Geometry: see drawing. Coordinates: mm, zero at the bounding-box minimum. Give positions to 0.01 mm unless a question says otherwise; leave off trailing zeros. Write each loop counter-clockwise with the first axis right and the second up, starting at its lowest first coordinate (ties: lowest second). Pieces come first, ordered by that corner, then holes.
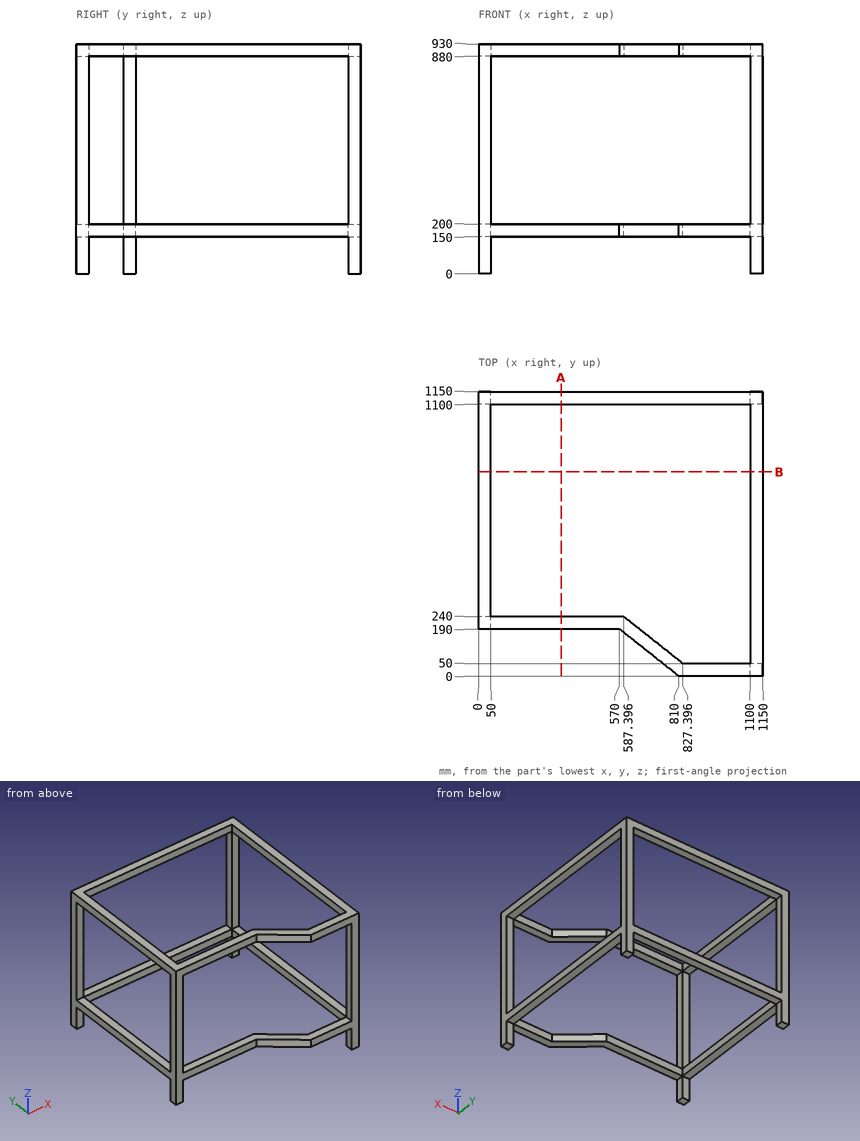
1. Line query: probe 1 along X at (y, z) = (209, 713); probe 2 along Y at (x, z) = (346, 172); probe 3 along Y at (x, z) = (624, 880.5). Output: solid intervals per line, ascending.
2. Pin query (flat end, axial travel): P1, Ø25, axis at x = 17, z = 79, coming from the -Y side. Return the tip coordinate at first contact, or that it passes through.
3. Section query B-B (y = 826.5). Return loops of the section in (x, z), plus the area to 3 significant figures.
4. Section query A-A (x = 334). Return loops of the section in (y, z).
The answers:
1. probe 1: x = 0 to 50
1. probe 2: y = 190 to 240, 1100 to 1150
1. probe 3: y = 147.25 to 211.02, 1100 to 1150
2. P1: stops at y = 190
3. outline: (0, 150) - (50, 150) - (50, 200) - (0, 200) - close; (0, 880) - (50, 880) - (50, 930) - (0, 930) - close; (1100, 150) - (1150, 150) - (1150, 200) - (1100, 200) - close; (1100, 880) - (1150, 880) - (1150, 930) - (1100, 930) - close
3. area: 10,000 mm2
4. outline: (190, 150) - (240, 150) - (240, 200) - (190, 200) - close; (190, 880) - (240, 880) - (240, 930) - (190, 930) - close; (1100, 150) - (1150, 150) - (1150, 200) - (1100, 200) - close; (1100, 880) - (1150, 880) - (1150, 930) - (1100, 930) - close
